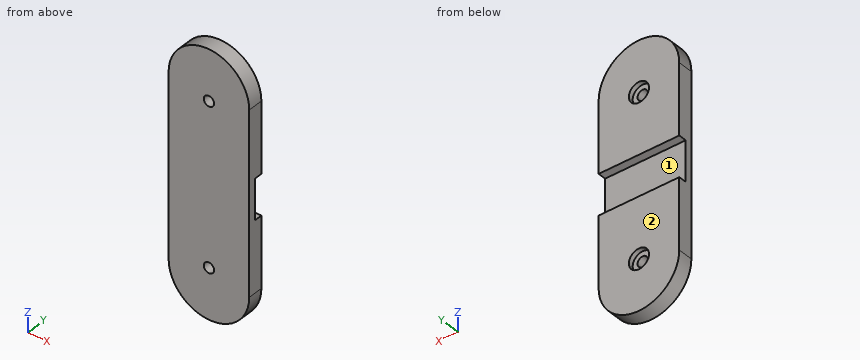
```python
from build123d import *

# Parameters (mm, degrees)
BOSS_EXTRUDE1_DEPTH                            = 4.7625
CBORE_FOR_4_BUTTON_HEAD_CAP_SCREW1_D           = 3.2639
CBORE_FOR_4_BUTTON_HEAD_CAP_SCREW1_CBORE_D     = 6.35
CBORE_FOR_4_BUTTON_HEAD_CAP_SCREW1_CBORE_DEPTH = 1.4986
SKETCH6_W                                      = 25.4
SKETCH6_H                                      = 12.7
CUT_EXTRUDE1_DEPTH                             = 2.54


with BuildPart() as part:
    # Sketch1 → Boss-Extrude1 (new body)
    with BuildSketch(Plane(origin=(0, 0, 0), x_dir=(1, 0, 0), z_dir=(0, 1, 0))):
        with BuildLine():
            Line((-12.7, -28.575), (-12.7, 28.575))
            ThreePointArc((-12.7, 28.575), (0, 41.275), (12.7, 28.575))
            Line((12.7, 28.575), (12.7, -28.575))
            ThreePointArc((12.7, -28.575), (0, -41.275), (-12.7, -28.575))
        make_face()
    extrude(amount=BOSS_EXTRUDE1_DEPTH)

    # CBORE for #4 Button Head Cap Screw1 (through all)
    with Locations(Plane(origin=(0, 4.7625, 0), x_dir=(-1, 0, 0), z_dir=(0, 1, 0))):
        with Locations((0, 25.4), (0, -25.4)):
            CounterBoreHole(CBORE_FOR_4_BUTTON_HEAD_CAP_SCREW1_D / 2, CBORE_FOR_4_BUTTON_HEAD_CAP_SCREW1_CBORE_D / 2, CBORE_FOR_4_BUTTON_HEAD_CAP_SCREW1_CBORE_DEPTH)

    # Sketch6 → Cut-Extrude1 (cut)
    with BuildSketch(Plane(origin=(0, 4.7625, 0), x_dir=(1, 0, 0), z_dir=(0, 1, 0))):
        Rectangle(SKETCH6_W, SKETCH6_H)
    extrude(amount=-CUT_EXTRUDE1_DEPTH, mode=Mode.SUBTRACT)


solid = part.part
```
Can you work these out from the model? Positions are in its coordinate system, mm. Face numbers are marked on the shaded views. A direction names the side the tool comes from. Coordinates: 2 decimals unless noted, no trailing zeros. Loops run counter-clockwise (first coordinate to the right, second up) from the corner with the lowest first, then second, coordinate; pieces in that order, holes last. Notation, with made-up numbers: M 10.5,-20 L 26.5,-20 A27 ccw 26.5,2 Z; hole C 56.25,45.25 d1. An arc over 180 degrees is marked long. Put each result on its own line as item: value. Start each with the question number.
(1) I need wall thicknesses on probe 1 along Z at (x, y) = (0, 0.75) (3 decimals); probe 2 along Z at (x, y) = (0, 2.3) (3 decimals); probe 3 along Y at (x, z) = (11.5, -6). Which ranges of each line are inside material? Lowest first, please.
(2) Which directions (+Z, -Z, +X, -X, +Y, -Y) give clear straight access to the entire face, cutting with the end or side of a thin tool? Please do the marked faces 1 and 2.
(3) Will these pins go through, and if not, where does the flat tip stop? pin 1 Ø3 at (x, z) = (1, -26.5) entering from +Y; pin 2 Ø0.8 at (x, y) = (4.5, 3.5) entering from +Z (3 decimals); pin 3 Ø4 at (x, z) = (-4, 3) entering from +Y.
(4) Imagine slicing it at C-C on x = -9.5. List the corners of the cut face in (y, z) for me, and give its area (3 significant figures).
(5) Imagine slicing it at A-A on x = 0. Give the number of separate pieces and of enclosed holes in the cut face, and give its area (3 significant figures).
(6) Imagine slicing it at D-D on z = 35.5. List the corners of the cut face in (x, y) for me, and give its area (3 significant figures).
(7) Imagine slicing it at B-B on z = -25.4. List the corners of the cut face in (x, y) for me (1 decimal), and give its area (3 significant figures).
Worked answers:
1. probe 1: z = -41.275 to -27.032, -23.768 to 23.768, 27.032 to 41.275
1. probe 2: z = -41.275 to -27.032, -23.768 to -6.35, 6.35 to 23.768, 27.032 to 41.275
1. probe 3: y = 0 to 2.22
2. face 1: +X, -X, +Y
2. face 2: +Z, -Z, +X, -X, +Y
3. pin 1: stops at y = 3.26
3. pin 2: stops at z = 40.595
3. pin 3: stops at y = 2.22
4. outline: M 0,-37 L 4.76,-37 L 4.76,-6.35 L 2.22,-6.35 L 2.22,6.35 L 4.76,6.35 L 4.76,37 L 0,37 Z
4. area: 320 mm2
5. separate pieces: 3
5. enclosed holes: 0
5. area: 321 mm2
6. outline: M -10.65,0 L 10.65,0 L 10.65,4.76 L -10.65,4.76 Z
6. area: 101 mm2
7. outline: M -12.7,0 L -1.6,0 L -1.6,3.3 L -3.2,3.3 L -3.2,4.8 L -12.7,4.8 Z; M 1.6,0 L 12.7,0 L 12.7,4.8 L 3.2,4.8 L 3.2,3.3 L 1.6,3.3 Z
7. area: 101 mm2
